Source: CAD feature listing. Evaluate the final solid. Frame: model axes, mm. Coordinates: 2 decimals unless noted, no trailing zeros. Loops run counter-clockwise (first coordinate to the right, second up) from the corner with the lowest first, then second, coordinate; pieces in that order, holes last. Notation, with made-up numbers: (17.5, 46) -> (37.5, 46) arc R30 ccw to (37.5, 81) -> close; hole circle Ø1 at (76, -9.75). An arc over 180 degrees is marked (long way). Answer as CSV lines item,"result".
from build123d import *

# Parameters (mm, degrees)
BOSS_EXTRUDE1_DEPTH = 6.35
SKETCH2_R           = 2.4892
CUT_EXTRUDE1_DEPTH  = 7.35


with BuildPart() as part:
    # Sketch1 → Boss-Extrude1 (new body)
    with BuildSketch(Plane.XY):
        Polygon((0, 0), (0, 120.65), (120.65, 120.65), (120.65, 41.91), (50.8, 41.91), (50.8, 0), align=None)
    extrude(amount=BOSS_EXTRUDE1_DEPTH)

    # Sketch2 → Cut-Extrude1 (cut, through all)
    with BuildSketch(Plane(origin=(0, 0, 0), x_dir=(-1, 0, 0), z_dir=(0, 0, -1))):
        with Locations((-110.49, 109.474)):
            Circle(SKETCH2_R)
        with Locations((-85.09, 109.474)):
            Circle(SKETCH2_R)
        with Locations((-85.09, 52.324)):
            Circle(SKETCH2_R)
        with Locations((-110.49, 52.324)):
            Circle(SKETCH2_R)
        with Locations((-38.1, 107.95)):
            Circle(SKETCH2_R)
        with Locations((-12.7, 107.95)):
            Circle(SKETCH2_R)
        with Locations((-12.7, 19.05)):
            Circle(SKETCH2_R)
        with Locations((-38.1, 19.05)):
            Circle(SKETCH2_R)
        with Locations((-38.1, 63.5)):
            Circle(SKETCH2_R)
        with Locations((-12.7, 63.5)):
            Circle(SKETCH2_R)
    extrude(amount=-CUT_EXTRUDE1_DEPTH, mode=Mode.SUBTRACT)


solid = part.part
(1) Material intervals for L1, parallel to Y at x = 12.7, z = 3; L2, parallel to Y at x = 85, z = 0.75; L3, parallel to Y at x = 36.5, z = 1.25, sorted ascending. Write a range as [from, to].
Computed values:
L1,"[0, 16.56], [21.54, 61.01], [65.99, 105.46], [110.44, 120.65]"
L2,"[41.91, 49.84], [54.81, 106.99], [111.96, 120.65]"
L3,"[0, 17.14], [20.96, 61.59], [65.41, 106.04], [109.86, 120.65]"
(2) Cut plane C-C (y = 63.5). Return the cut outline in (x, z).
Computed values:
outline,"(0, 0) -> (10.21, 0) -> (10.21, 6.35) -> (0, 6.35) -> close; (15.19, 0) -> (35.61, 0) -> (35.61, 6.35) -> (15.19, 6.35) -> close; (40.59, 0) -> (120.65, 0) -> (120.65, 6.35) -> (40.59, 6.35) -> close"
(3) Cut plane D-D (z = 2). State how many separate pieces and enclosed holes the cut face has, then the cut area to 3 significant figures.
Computed values:
separate pieces,"1"
enclosed holes,"10"
area,"11,400 mm^2"
(4) Cut plane B-B (x = 85.09). Return the cut outline in (y, z).
Computed values:
outline,"(41.91, 0) -> (49.83, 0) -> (49.83, 6.35) -> (41.91, 6.35) -> close; (54.81, 0) -> (106.98, 0) -> (106.98, 6.35) -> (54.81, 6.35) -> close; (111.96, 0) -> (120.65, 0) -> (120.65, 6.35) -> (111.96, 6.35) -> close"
(5) Draft query along Y for faces 1 (the flat face through (50.8, 21, 3)), 2 (the cylindrical face through (86.92, 111.16, 3.13)), 3 (the flat face through (86, 41.91, 3)). Return one class per face: released by +Y, released by -Y, zero draft, split by the parting line, or undercut.
Computed values:
face 1,"zero draft"
face 2,"undercut"
face 3,"released by -Y"
(6) Cut plane A-A (x = 38.1). Return the cut outline in (y, z), then the cut area to 3 significant figures.
Computed values:
outline,"(0, 0) -> (16.56, 0) -> (16.56, 6.35) -> (0, 6.35) -> close; (21.54, 0) -> (61.01, 0) -> (61.01, 6.35) -> (21.54, 6.35) -> close; (65.99, 0) -> (105.46, 0) -> (105.46, 6.35) -> (65.99, 6.35) -> close; (110.44, 0) -> (120.65, 0) -> (120.65, 6.35) -> (110.44, 6.35) -> close"
area,"671 mm^2"
(7) Pin query (flat end, axial travel): pin 1 Ø1.9 at (x, z) = (87, 2.5) entering from -Y; pin 2 Ø3 at (y, z) = (15.5, 4.5) entering from +X. Return the tip coordinate at first contact, or that it passes through.
Computed values:
pin 1,"y = 41.91"
pin 2,"x = 50.8"
